Check sheet for the drawn part. Datum: minimum x, y, z corner. Units: mm. Coordinates: 2 decimals unless noted, no trailing zeros. Write each loop counter-clockwise with the first axis right and the second up, starting at its lowest first coordinate (ties: lowest second). Pieces come first, ordered by that corner, then holes. Notation, with made-up numbers: (-8, 53.25) -> (4, 53.25) arc R34 ccw to (4, 92.25) -> close; hole circle Ø4 at (54, -30). An arc over 180 degrees is marked (long way). Write item = value, one per line. Start each with the question number.
(1) Section check C-C (y = 2.25). Record the cut outline in (x, z).
(2) Mould release check, pull along X, two halves, no side actions. Record for the marked faces 1, 2 and 3: released by +X, released by -X, zero draft, split by the parting line, or undercut.
(3) Material ranges on probe 1 along X at (y, z) = (2.2, 16); probe 2 along Z at (x, y) = (8, 2.2); probe 3 along X at (y, z) = (3.5, 14), recorded low to high. Write a range as [from, to].
(4) Section check B-B (z = 16). Record the cut outline in (x, y).
(5) Section check A-A (x = 8). Record the cut outline in (y, z), plus the area to 3 significant figures.
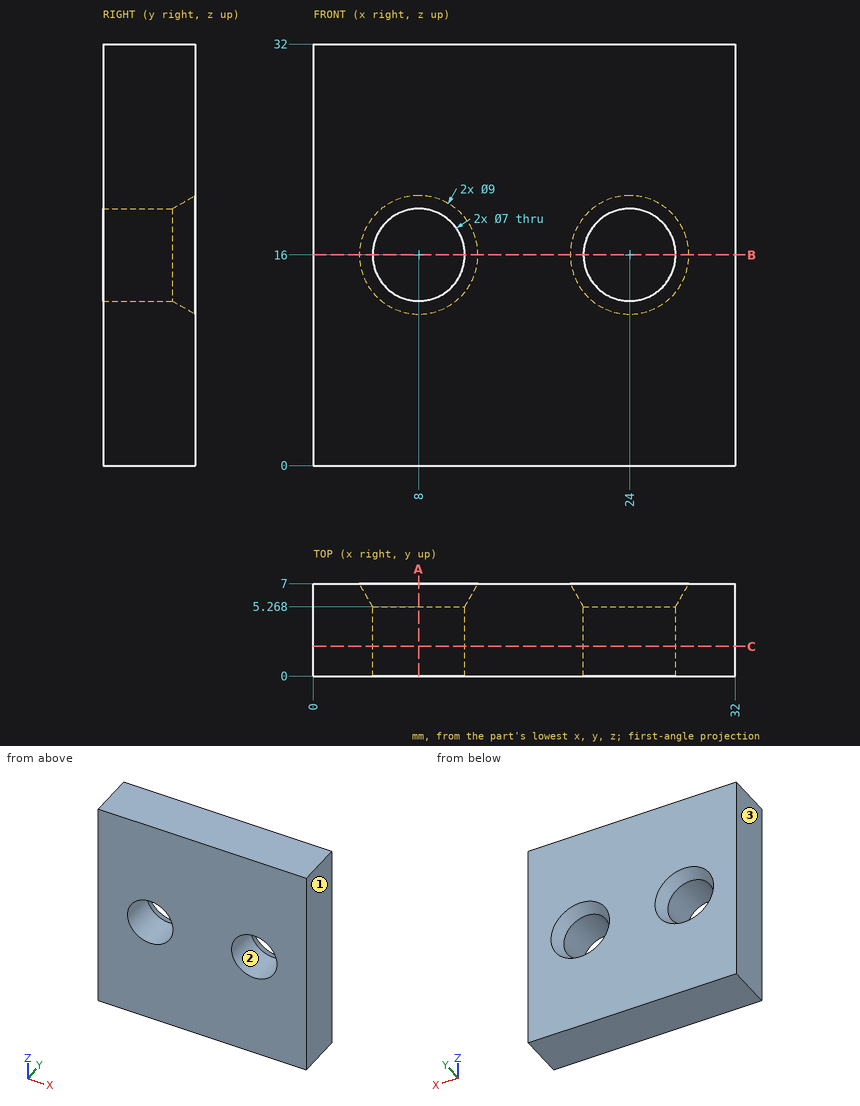
Response:
q1.outline = (0, 0) -> (32, 0) -> (32, 32) -> (0, 32) -> close; hole circle Ø7 at (8, 16); hole circle Ø7 at (24, 16)
q2.face_1 = released by +X
q2.face_2 = undercut
q2.face_3 = released by -X
q3.probe_1 = [0, 4.5], [11.5, 20.5], [27.5, 32]
q3.probe_2 = [0, 12.5], [19.5, 32]
q3.probe_3 = [0, 5.13], [10.87, 21.13], [26.87, 32]
q4.outline = (0, 0) -> (4.5, 0) -> (4.5, 5.27) -> (3.5, 7) -> (0, 7) -> close; (11.5, 0) -> (20.5, 0) -> (20.5, 5.27) -> (19.5, 7) -> (12.5, 7) -> (11.5, 5.27) -> close; (27.5, 0) -> (32, 0) -> (32, 7) -> (28.5, 7) -> (27.5, 5.27) -> close
q5.outline = (0, 0) -> (7, 0) -> (7, 11.5) -> (5.27, 12.5) -> (0, 12.5) -> close; (0, 19.5) -> (5.27, 19.5) -> (7, 20.5) -> (7, 32) -> (0, 32) -> close
q5.area = 173 mm2
